Verification items for the finished model (mm, model axes). A direction names the side the tool comes from. Coordinates: 2 decimals unless noted, no trailing zeros. Loops run counter-clockwise (first coordinate to the right, second up) from the corner with the lowest first, then second, coordinate; pieces in that order, holes last.
Q1. Go/stop test with flat-tipped pins: P1, Ø1.5, axis at x = 14.5, y = -42, coming from the -Z side; P2, Ø1, axis at x = 21, y = -30.5, coming from the +Z side; P3, Ø6, axis at x = 6, z = 7.5, coming from the +Y side. Record where each tip stops, or that it passes through.
Q2. Sectioned sample at B-B (y = -42). Enter the section's corners in (x, z) (3 decimals), then the cut area to 3 significant figures.
Q3. Access from +Z, -Z, +X, -X, +Y, -Y to the whole of each face (thin tool, end or side, straight path). Record for faces 4 (the face through (43.462, -66.406, 8.566)), 5 (the face through (46.1, -37.2, 14.8)), 6 (the face through (43.462, -17.084, 8.566)), 7 (the face through (4, -43, 5)).
Q4. Sectioned sample at D-D (y = -18). Enter the section's corners in (x, z).
Q5. Mould release check, pull along X, two halves, no side actions. Record for faces 1 (the face through (26.72, -49.19, 9.86)), 2 (the face through (50, -41, 2)), 3 (the face through (19, -41, 0)): +X half, -X half, draft (parallel to the pull), parting line (faces both ways), or undercut.
Q6. Sectioned sample at A-A (x = 32). Enter the section's corners in (y, z), then the cut area to 3 significant figures.
Q7. Sectioned sample at C-C (z = 2.75). Enter the section's corners in (x, y), then the cut area to 3 significant figures.
Q8. Material ranges on probe 1 along Z at (x, y) = (15, -38); probe 2 along X at (y, z) = (-43.5, 5); probe 3 along X at (y, z) = (-44.5, 8.5), recorded low to high.
Autodesk Inventor part; units mm, degrees
ref_plane "YZ Plane" through (0, 0, 0) normal (1, 0, 0) x (0, 1, 0)
ref_plane "XZ Plane" through (0, 0, 0) normal (0, 1, 0) x (-1, 0, 0)
ref_plane "XY Plane" through (0, 0, 0) normal (0, 0, 1) x (1, 0, 0)
sketch "Sketch1" plane through (0, 0, 0) normal (0, 0, 1) x (1, 0, 0)
  line L0 (0, 0) -> (50, 0)
  line L1 (50, 0) -> (50, -84)
  line L2 (50, -84) -> (0, -84)
  line L3 (0, -84) -> (0, 0)
  circle A0 centre (34.5628, -42) radius 12.4978
  circle A1 centre (34.5628, -42) radius 10.6396
  dimension "d0" = 50
  dimension "d1" = 84
extrude "Extrusion1" add sketch "Sketch1" along normal blind 10 contours L0 L1 L2 L3
extrude "Extrusion2" add sketch "Sketch1" along normal blind 20 contours A0
chamfer "Chamfer1" distance 6 angle 45 1 edges at (50, -42, 10)
chamfer "Chamfer2" distance 4 angle 45 2 edges at (44, -67.0968, 10) (44, -16.9032, 10)
chamfer "Chamfer3" distance 9 angle 45 1 edges at (0, -42, 10)
chamfer "Chamfer4" distance 6 angle 45 2 edges at (24.5, 0, 10) (24.5, -84, 10)
equation "\"BendRadius\" = Thickness"
equation "\"BendReliefWidth\" = Thickness"
equation "\"BendReliefDepth\" = 0.5 * Thickness"
equation "\"CornerReliefSize\" = 4 * Thickness"
equation "\"MinimumRemnant\" = 2 * Thickness"
equation "\"TransitionRadius\" = BendRadius"
equation "\"JacobiRadiusSize\" = BendRadius"
equation "\"GapSize\" = Thickness"
Geometry check:
1. P1: stops at z = 0
1. P2: stops at z = 10
1. P3: stops at y = -0.5
2. outline: (0, 0) - (23.923, 0) - (23.923, 20) - (22.065, 20) - (22.065, 10) - (9, 10) - (0, 1) - close; (45.202, 0) - (50, 0) - (50, 4) - (47.061, 6.939) - (47.061, 20) - (45.202, 20) - close
2. area: 271 mm2
3. face 4: +Z, +X, -Y
3. face 5: +Z
3. face 6: +Z, +X, +Y
3. face 7: +Z, -X, +Y, -Y
4. outline: (0, 0) - (50, 0) - (50, 4) - (46.83, 7.17) - (40, 10) - (9, 10) - (0, 1) - close
5. face 1: undercut
5. face 2: +X half
5. face 3: draft
6. outline: (-84, 0) - (-52.33, 0) - (-52.33, 20) - (-54.23, 20) - (-54.23, 10) - (-78, 10) - (-84, 4) - close; (-31.67, 0) - (0, 0) - (0, 4) - (-6, 10) - (-29.77, 10) - (-29.77, 20) - (-31.67, 20) - close
6. area: 636 mm2
7. outline: (1.75, -84) - (50, -84) - (50, 0) - (1.75, 0) - close; hole circle Ø21.28 at (34.56, -42)
7. area: 3,700 mm2
8. probe 1: z = 0 to 10
8. probe 2: x = 4 to 24.03, 45.1 to 49
8. probe 3: x = 7.5 to 24.22, 44.9 to 46.81
